from build123d import *

# Parameters (mm, degrees)
F0_R      = 1.016
F0_W      = 62.484
F0_H      = 5.1308
F0_W_2    = 5.842
F0_H_2    = 5.842
F0_W_3    = 6.604
F0_H_3    = 11.6078
F0_W_4    = 4.064
F0_H_4    = 10.414
F0_W_5    = 12.8016
F0_H_5    = 12.319
F0_W_6    = 8.1788
F0_H_6    = 7.6962
F0_W_7    = 8.382
F0_H_7    = 14.986
F0_W_8    = 12.446
F0_H_8    = 6.096
F1_DEPTH  = 1.524
F2_DEPTH  = 8.382
F0_W_9    = 0.762
F3_DEPTH  = 6.35
F4_DEPTH  = 4.826
F5_DEPTH  = 2.286
F0_W_10   = 2.5908
F6_DEPTH  = 1.27
F0_W_11   = 0.889
F7_DEPTH  = 3.81
F8_DEPTH  = 4.572
F9_DEPTH  = 0.762
F11_DEPTH = 1.778


with BuildPart() as f1:
    # F0 (on Top) → F1 (new body)
    with BuildSketch(Plane.XY):
        Polygon((38.1, 26.035), (-38.1, 26.035), (-38.1, 21.463), (-29.718, 21.463), (-29.718, 6.477), (-38.1, 6.477), (-38.1, 3.175), (-25.654, 3.175), (-25.654, -2.921), (-38.1, -2.921), (-38.1, -5.969), (-29.718, -5.969), (-29.718, -20.955), (-38.1, -20.955), (-38.1, -26.035), (38.1, -26.035), (38.1, -4.445), (29.9212, -4.445), (29.9212, 3.2512), (38.1, 3.2512), (38.1, 7.3152), (25.2984, 7.3152), (25.2984, 19.6342), (38.1, 19.6342), align=None)
        with Locations((-32.385, -22.86)):
            Circle(F0_R, mode=Mode.SUBTRACT)
        with Locations((2.032, -22.8346)):
            Rectangle(F0_W, F0_H, mode=Mode.SUBTRACT)
        with Locations((3.429, -14.605)):
            Rectangle(F0_W_2, F0_H_2, mode=Mode.SUBTRACT)
        with Locations((34.544, -22.86)):
            Circle(F0_R, mode=Mode.SUBTRACT)
        with Locations((33.02, -14.0589)):
            Rectangle(F0_W_3, F0_H_3, mode=Mode.SUBTRACT)
        with Locations((-32.385, 23.114)):
            Circle(F0_R, mode=Mode.SUBTRACT)
        with Locations((22.098, 11.43)):
            Rectangle(F0_W_4, F0_H_4, mode=Mode.SUBTRACT)
        with Locations((2.032, 22.8346)):
            Rectangle(F0_W, F0_H, mode=Mode.SUBTRACT)
        with Locations((34.671, 23.241)):
            Circle(F0_R, mode=Mode.SUBTRACT)
        with Locations((2.032, 22.8346)):
            Rectangle(F0_W, F0_H)
        with Locations((31.6992, 13.4747)):
            Rectangle(F0_W_5, F0_H_5)
        with Locations((34.0106, -0.5969)):
            Rectangle(F0_W_6, F0_H_6)
        with Locations((33.02, -14.0589)):
            Rectangle(F0_W_3, F0_H_3)
        with Locations((2.032, -22.8346)):
            Rectangle(F0_W, F0_H)
        with Locations((3.429, -14.605)):
            Rectangle(F0_W_2, F0_H_2)
        with Locations((-33.909, -13.462)):
            Rectangle(F0_W_7, F0_H_7)
        with Locations((-31.877, 0.127)):
            Rectangle(F0_W_8, F0_H_8)
        with Locations((-33.909, 13.97)):
            Rectangle(F0_W_7, F0_H_7)
        with Locations((22.098, 11.43)):
            Rectangle(F0_W_4, F0_H_4)
    extrude(amount=-F1_DEPTH)

    # F0 (on Top) → F2 (join)
    with BuildSketch(Plane.XY):
        with Locations((2.032, 22.8346)):
            Rectangle(F0_W, F0_H)
        with Locations((2.032, -22.8346)):
            Rectangle(F0_W, F0_H)
    extrude(amount=F2_DEPTH)

    # F0 (on Top) → F3 (join)
    with BuildSketch(Plane.XY):
        with Locations((-33.909, 13.97)):
            Rectangle(F0_W_7, F0_H_7)
        with Locations((-38.481, 13.97)):
            Rectangle(F0_W_9, F0_H_7)
        with Locations((-38.481, -13.462)):
            Rectangle(F0_W_9, F0_H_7)
        with Locations((-33.909, -13.462)):
            Rectangle(F0_W_7, F0_H_7)
    extrude(amount=F3_DEPTH)

    # F0 (on Top) → F4 (join)
    with BuildSketch(Plane.XY):
        with Locations((-31.877, 0.127)):
            Rectangle(F0_W_8, F0_H_8)
    extrude(amount=F4_DEPTH)

    # F0 (on Top) → F5 (join)
    with BuildSketch(Plane.XY):
        with Locations((3.429, -14.605)):
            Rectangle(F0_W_2, F0_H_2)
    extrude(amount=F5_DEPTH)

    # F0 (on Top) → F6 (join)
    with BuildSketch(Plane.XY):
        with Locations((31.6992, 13.4747)):
            Rectangle(F0_W_5, F0_H_5)
        with Locations((39.3954, 13.4747)):
            Rectangle(F0_W_10, F0_H_5)
    extrude(amount=F6_DEPTH)

    # F0 (on Top) → F7 (join)
    with BuildSketch(Plane.XY):
        with Locations((34.0106, -0.5969)):
            Rectangle(F0_W_6, F0_H_6)
        with Locations((38.5445, -0.5969)):
            Rectangle(F0_W_11, F0_H_6)
    extrude(amount=F7_DEPTH)

    # F0 (on Top) → F8 (join)
    with BuildSketch(Plane.XY):
        with Locations((33.02, -14.0589)):
            Rectangle(F0_W_3, F0_H_3)
    extrude(amount=F8_DEPTH)

    # F0 (on Top) → F9 (join)
    with BuildSketch(Plane.XY):
        with Locations((22.098, 11.43)):
            Rectangle(F0_W_4, F0_H_4)
    extrude(amount=F9_DEPTH)

    # F10 (on face) → F11 (join)
    with BuildSketch(Plane(origin=(-38.1, 0, 0), x_dir=(0, -1, 0), z_dir=(-1, 0, 0))):
        with BuildLine():
            Line((-0.127, 2.286), (2.413, 2.286))
            ThreePointArc((2.413, 2.286), (1.669051, 4.082051), (-0.127, 4.826))
            Line((-0.127, 4.826), (-0.127, 2.286))
        make_face()
        with BuildLine():
            Line((-0.127, 2.286), (-0.127, 4.826))
            ThreePointArc((-0.127, 4.826), (-1.923051, 4.082051), (-2.667, 2.286))
            Line((-2.667, 2.286), (-0.127, 2.286))
        make_face()
        with BuildLine():
            ThreePointArc((-2.667, 2.286), (-0.127, -0.254), (2.413, 2.286))
            Line((2.413, 2.286), (-0.127, 2.286))
            Line((-0.127, 2.286), (-2.667, 2.286))
        make_face()
    extrude(amount=F11_DEPTH)


solid = f1.part
Source: CAD feature listing. Evaluate the final solid. Frame: model axes, mm. A direction names the side the tool comes from. Give positions to 0.01 mm unless a question says otherwise; leave off trailing zeros. Write each loop counter-clockwise with the first axis right and the second up, starting at its lowest first coordinate (ties: lowest second). Pieces come first, ordered by that corner, then holes. Notation, with made-up numbers: (77.5, 12.5) - (136.5, 12.5) arc R16 ccw to (136.5, 27.5) - close; hole circle Ø10 at (15, -25.5). An arc over 180 degrees is marked (long way). Write item = value, one per line. Start each with the question number.
Q1. Material intervals for probe 1 along X at (y, z) = (-16, 0.5); probe 2 along Y at (x, z) = (-32.5, 2.75) (3 decimals); probe 3 along Y at (x, z) = (31.5, 3.75) (3 decimals), sorted ascending.
Q2. Cut plane C-C, the plane y = 12. Return loops of the section in (x, z).
Q3. Reachability of faces 5 (the flat face through (3, -11.684, 1)), 6 (the flat face through (-34, -5.969, 3)), 7 (the flat face through (2, 25.4, 4)), 8 (the flat face through (39, 14, 0)) from +Z, -Z, +X, -X, +Y, -Y: full face, straight path, thin tool, end or side. Return the list, or none.
Q4. Cut plane B-B, the plane x = 5.5. Return loops of the section in (y, z) (3 decimals).
Q5. Draft query along Y for faces 1 (the flat face through (1, 26.035, -1)), 2 (the flat face through (2, -25.4, 4)), 3 (the flat face through (-39.878, 0, 2)), 4 (the flat face through (-25.654, 0, 2)). Return one class per face: +Y half, -Y half, draft (parallel to the pull), parting line (faces both ways), or undercut.
Q6. Cut plane A-A, the plane y = -22.86. Return loops of the section in (x, z).
Q7. Pin query (flat end, axial travel): pin 1 Ø12 at (x, y) = (-27, -10.5) entering from +Z; pin 2 Ø1.4 at (x, z) = (31, 0.5) entering from -Y (3 decimals); pin 3 Ø2.5 at (x, y) = (35.5, -2) entering from +Z; pin 4 Ø1 at (y, z) = (11, 1) entering from -X. Return the tip coordinate at first contact, or that it passes through.
Q8. Cut plane D-D, the plane y = 17.5. Return loops of the section in (x, z).
Computed values:
q1.probe_1 = -38.86 to -29.72, 0.51 to 6.35, 29.72 to 36.32
q1.probe_2 = -20.955 to -5.969, -2.921 to 3.175, 6.477 to 21.463
q1.probe_3 = -25.4 to -20.269, -19.863 to -8.255, -4.445 to 3.251, 20.269 to 25.4
q2.outline = (-38.86, 0) - (-38.1, 0) - (-38.1, -1.52) - (38.1, -1.52) - (38.1, 0) - (40.69, 0) - (40.69, 1.27) - (25.3, 1.27) - (25.3, 0) - (24.13, 0) - (24.13, 0.76) - (20.07, 0.76) - (20.07, 0) - (-29.72, 0) - (-29.72, 6.35) - (-38.86, 6.35) - close
q3.face_5 = +Z
q3.face_6 = +Z, +X, -X
q3.face_7 = +Z, +X, -X, +Y
q3.face_8 = -Z, +X, +Y, -Y
q4.outline = (-26.035, -1.524) - (26.035, -1.524) - (26.035, 0) - (25.4, 0) - (25.4, 8.382) - (20.269, 8.382) - (20.269, 0) - (-11.684, 0) - (-11.684, 2.286) - (-17.526, 2.286) - (-17.526, 0) - (-20.269, 0) - (-20.269, 8.382) - (-25.4, 8.382) - (-25.4, 0) - (-26.035, 0) - close
q5.face_1 = +Y half
q5.face_2 = -Y half
q5.face_3 = draft
q5.face_4 = undercut
q6.outline = (-38.1, -1.52) - (-33.4, -1.52) - (-33.4, 0) - (-38.1, 0) - close; (-31.37, -1.52) - (33.53, -1.52) - (33.53, 0) - (33.27, 0) - (33.27, 8.38) - (-29.21, 8.38) - (-29.21, 0) - (-31.37, 0) - close; (35.56, -1.52) - (38.1, -1.52) - (38.1, 0) - (35.56, 0) - close
q7.pin_1 = 6.35
q7.pin_2 = -26.035
q7.pin_3 = 3.81
q7.pin_4 = -38.86
q8.outline = (-38.86, 0) - (-38.1, 0) - (-38.1, -1.52) - (38.1, -1.52) - (38.1, 0) - (40.69, 0) - (40.69, 1.27) - (25.3, 1.27) - (25.3, 0) - (-29.72, 0) - (-29.72, 6.35) - (-38.86, 6.35) - close
